from build123d import *

# Parameters (mm, degrees)
SKETCH1_R               = 8
SKETCH1_R_2             = 6
BOSS_EXTRUDE1_DEPTH     = 170
SKETCH2_W               = 50
SKETCH2_H               = 2.5
CUT_EXTRUDE1_DEPTH      = 9
CUT_EXTRUDE1_DEPTH_BACK = 9


with BuildPart() as part:
    # Sketch1 → Boss-Extrude1 (new body, symmetric)
    with BuildSketch(Plane(origin=(0, 0, 0), x_dir=(0, 0, -1), z_dir=(1, 0, 0))):
        Circle(SKETCH1_R)
        Circle(SKETCH1_R_2, mode=Mode.SUBTRACT)
    extrude(amount=BOSS_EXTRUDE1_DEPTH, both=True)

    # Sketch2 → Cut-Extrude1 (cut, two sides)
    with BuildSketch(Plane.XY) as cut_extrude1_sk:
        with Locations((145, 0)):
            Rectangle(SKETCH2_W, SKETCH2_H)
    extrude(amount=CUT_EXTRUDE1_DEPTH, mode=Mode.SUBTRACT)
    extrude(cut_extrude1_sk.sketch, amount=-CUT_EXTRUDE1_DEPTH_BACK, mode=Mode.SUBTRACT)


solid = part.part
Geometry: final body of the model. Coordinates: model frame, mm. Give positions to 0.01 mm unless a question says otherwise; leave off trailing zeros. Loops run counter-clockwise (first coordinate to the right, second up) from the corner with the lowest first, then second, coordinate; pieces in that order, holes last. Notation, with made-up numbers: (45.25, 5.5) - (84.25, 5.5) arc R26 ccw to (84.25, 27.5) - close; hole circle Ø1 at (20.25, 45.5). An arc over 180 degrees is marked (long way). One line per question, with ' | ' between items. Start each with the question number.
(1) Contact query for flat-ended pins moving along their axis: pin 1 (6 mm diameter, centred on x = -28, y = 5.5, fed in from +Z); pin 2 (0.6 mm diameter, centred on y = -0.5, z = -6.5, fed in from +X); pin 3 (1 mm diameter, centred on x = 150.5, z = 7, fed in from +Y); pin 4 (2 mm diameter, centred on y = -3, z = 1.5, fed in from -X). Output: stop coordinate, or through.
(2) Ray query, line 1 (Y direction, x = -15, z = 1); line 2 (Y direction, x = -6, z = 0); line 3 (Z direction, x = -32.5, y = 3.25). Return the intervals inside material, ascending. Write a range as from..to.
(3) Pull-direction query (Z, two-part tool) for faces 1 (the flat face through (170, 6.2, 0.1)), 2 (the cylindrical face through (-2.38, 1.802, -5.723)), 3 (the cylindrical face through (2.38, -3.06, -7.39)); classes: released by +Z, released by -Z, zero draft, split by the parting line, or undercut.
(4) Section query A-A on z = 3. Return loops of the section in (x, y), then the cut area to 3 significant figures.
(5) Section query B-B on x = -110. Return loops of the section in (y, z), then the cut area to 3 significant figures.
The answers:
1) pin 1: z = 7.6 | pin 2: x = 120 | pin 3: y = 4.66 | pin 4: through
2) line 1: -7.94..-5.92, 5.92..7.94 | line 2: -8..-6, 6..8 | line 3: -7.31..-5.04, 5.04..7.31
3) face 1: zero draft | face 2: undercut | face 3: split by the parting line
4) outline: (-170, -7.42) - (170, -7.42) - (170, -5.2) - (-170, -5.2) - close; (-170, 5.2) - (170, 5.2) - (170, 7.42) - (-170, 7.42) - close | area: 1,510 mm2
5) outline: circle Ø16 at (0, 0); hole circle Ø12 at (0, 0) | area: 88.0 mm2
